from build123d import *

# Parameters (mm, degrees)
BOSS_EXTRUDE1_DEPTH = 5
SKETCH2_W           = 55
SKETCH2_H           = 50
CUT_EXTRUDE1_DEPTH  = 273.349040755
CUT_EXTRUDE2_DEPTH  = 273.349040755
SKETCH4_W           = 30
SKETCH4_H           = 1
CUT_EXTRUDE3_DEPTH  = 273.349040755
CUT_EXTRUDE4_DEPTH  = 273.349040755
CUT_EXTRUDE5_DEPTH  = 273.349040755
CUT_EXTRUDE6_DEPTH  = 273.349040755


with BuildPart() as part:
    # Sketch1 → Boss-Extrude1 (new body)
    with BuildSketch(Plane(origin=(0, 0, 0), x_dir=(1, 0, 0), z_dir=(0, 1, 0))):
        Polygon((0, 0), (0, -43), (30, -43), (30, -48), (0, -48), (0, -73), (90, -73), (90, 257), (-55, 257), (-55, 5), (0, 5), (30, 5), (30, 0), align=None)
    extrude(amount=BOSS_EXTRUDE1_DEPTH)

    # Sketch2 → Cut-Extrude1 (cut, through all)
    with BuildSketch(Plane(origin=(0, 5, 0), x_dir=(1, 0, 0), z_dir=(0, 1, 0))):
        with Locations((-27.5, 232)):
            Rectangle(SKETCH2_W, SKETCH2_H)
    extrude(amount=-CUT_EXTRUDE1_DEPTH, mode=Mode.SUBTRACT)

    # Sketch3 → Cut-Extrude2 (cut, through all)
    with BuildSketch(Plane(origin=(0, 5, 0), x_dir=(1, 0, 0), z_dir=(0, 1, 0))):
        with BuildLine():
            Line((66, 237), (66, 157))
            ThreePointArc((66, 157), (64, 155), (62, 157))
            Line((62, 157), (62, 237))
            ThreePointArc((62, 237), (64, 239), (66, 237))
        make_face()
        with BuildLine():
            Line((66, 127), (66, 47))
            ThreePointArc((66, 47), (64, 45), (62, 47))
            Line((62, 47), (62, 127))
            ThreePointArc((62, 127), (64, 129), (66, 127))
        make_face()
        with BuildLine():
            Line((66, 17), (66, -63))
            ThreePointArc((66, -63), (64, -65), (62, -63))
            Line((62, -63), (62, 17))
            ThreePointArc((62, 17), (64, 19), (66, 17))
        make_face()
        with BuildLine():
            Line((8, 237), (8, 157))
            ThreePointArc((8, 157), (10, 155), (12, 157))
            Line((12, 157), (12, 237))
            ThreePointArc((12, 237), (10, 239), (8, 237))
        make_face()
        with BuildLine():
            Line((8, 127), (8, 47))
            ThreePointArc((8, 47), (10, 45), (12, 47))
            Line((12, 47), (12, 127))
            ThreePointArc((12, 127), (10, 129), (8, 127))
        make_face()
    extrude(amount=-CUT_EXTRUDE2_DEPTH, mode=Mode.SUBTRACT)

    # Sketch4 → Cut-Extrude3 (cut, through all)
    with BuildSketch(Plane(origin=(0, 5, 0), x_dir=(1, 0, 0), z_dir=(0, 1, 0))):
        with Locations((15, -0.5)):
            Rectangle(SKETCH4_W, SKETCH4_H)
        with Locations((15, -42.5)):
            Rectangle(SKETCH4_W, SKETCH4_H)
    extrude(amount=-CUT_EXTRUDE3_DEPTH, mode=Mode.SUBTRACT)

    # Sketch5 → Cut-Extrude4 (cut, through all)
    with BuildSketch(Plane(origin=(0, 5, 0), x_dir=(1, 0, 0), z_dir=(0, 1, 0))):
        with BuildLine():
            Line((6, -19.5), (46, -19.5))
            ThreePointArc((46, -19.5), (48, -21.5), (46, -23.5))
            Line((46, -23.5), (6, -23.5))
            ThreePointArc((6, -23.5), (4, -21.5), (6, -19.5))
        make_face()
        with BuildLine():
            Line((6, -3.5), (46, -3.5))
            ThreePointArc((46, -3.5), (48, -5.5), (46, -7.5))
            Line((46, -7.5), (6, -7.5))
            ThreePointArc((6, -7.5), (4, -5.5), (6, -3.5))
        make_face()
        with BuildLine():
            Line((6, -35.5), (46, -35.5))
            ThreePointArc((46, -35.5), (48, -37.5), (46, -39.5))
            Line((46, -39.5), (6, -39.5))
            ThreePointArc((6, -39.5), (4, -37.5), (6, -35.5))
        make_face()
    extrude(amount=-CUT_EXTRUDE4_DEPTH, mode=Mode.SUBTRACT)

    # Sketch6 → Cut-Extrude5 (cut, through all)
    with BuildSketch(Plane(origin=(0, 5, 0), x_dir=(1, 0, 0), z_dir=(0, 1, 0))):
        with BuildLine():
            Line((-43, 197), (-43, 157))
            ThreePointArc((-43, 157), (-45, 155), (-47, 157))
            Line((-47, 157), (-47, 197))
            ThreePointArc((-47, 197), (-45, 199), (-43, 197))
        make_face()
        with BuildLine():
            Line((-33, 197), (-33, 157))
            ThreePointArc((-33, 157), (-35, 155), (-37, 157))
            Line((-37, 157), (-37, 197))
            ThreePointArc((-37, 197), (-35, 199), (-33, 197))
        make_face()
        with BuildLine():
            Line((-23, 197), (-23, 157))
            ThreePointArc((-23, 157), (-25, 155), (-27, 157))
            Line((-27, 157), (-27, 197))
            ThreePointArc((-27, 197), (-25, 199), (-23, 197))
        make_face()
        with BuildLine():
            Line((-13, 197), (-13, 157))
            ThreePointArc((-13, 157), (-15, 155), (-17, 157))
            Line((-17, 157), (-17, 197))
            ThreePointArc((-17, 197), (-15, 199), (-13, 197))
        make_face()
        with BuildLine():
            Line((-3, 197), (-3, 157))
            ThreePointArc((-3, 157), (-5, 155), (-7, 157))
            Line((-7, 157), (-7, 197))
            ThreePointArc((-7, 197), (-5, 199), (-3, 197))
        make_face()
        with BuildLine():
            Line((-43, 15), (-43, 55))
            ThreePointArc((-43, 55), (-45, 57), (-47, 55))
            Line((-47, 55), (-47, 15))
            ThreePointArc((-47, 15), (-45, 13), (-43, 15))
        make_face()
        with BuildLine():
            Line((-33, 15), (-33, 55))
            ThreePointArc((-33, 55), (-35, 57), (-37, 55))
            Line((-37, 55), (-37, 15))
            ThreePointArc((-37, 15), (-35, 13), (-33, 15))
        make_face()
        with BuildLine():
            Line((-23, 15), (-23, 55))
            ThreePointArc((-23, 55), (-25, 57), (-27, 55))
            Line((-27, 55), (-27, 15))
            ThreePointArc((-27, 15), (-25, 13), (-23, 15))
        make_face()
        with BuildLine():
            Line((-13, 15), (-13, 55))
            ThreePointArc((-13, 55), (-15, 57), (-17, 55))
            Line((-17, 55), (-17, 15))
            ThreePointArc((-17, 15), (-15, 13), (-13, 15))
        make_face()
        with BuildLine():
            Line((-3, 15), (-3, 55))
            ThreePointArc((-3, 55), (-5, 57), (-7, 55))
            Line((-7, 55), (-7, 15))
            ThreePointArc((-7, 15), (-5, 13), (-3, 15))
        make_face()
    extrude(amount=-CUT_EXTRUDE5_DEPTH, mode=Mode.SUBTRACT)

    # Sketch7 → Cut-Extrude6 (cut, through all)
    with BuildSketch(Plane(origin=(0, 5, 0), x_dir=(1, 0, 0), z_dir=(0, 1, 0))):
        with BuildLine():
            Line((-44.604932944, 139), (-5, 139))
            ThreePointArc((-5, 139), (-3, 137), (-5, 135))
            Line((-5, 135), (-44.604932944, 135))
            ThreePointArc((-44.604932944, 135), (-46.604932944, 137), (-44.604932944, 139))
        make_face()
        with BuildLine():
            Line((-44.604932944, 119), (-5, 119))
            ThreePointArc((-5, 119), (-3, 117), (-5, 115))
            Line((-5, 115), (-44.604932944, 115))
            ThreePointArc((-44.604932944, 115), (-46.604932944, 117), (-44.604932944, 119))
        make_face()
        with BuildLine():
            Line((-44.604932944, 99), (-5, 99))
            ThreePointArc((-5, 99), (-3, 97), (-5, 95))
            Line((-5, 95), (-44.604932944, 95))
            ThreePointArc((-44.604932944, 95), (-46.604932944, 97), (-44.604932944, 99))
        make_face()
        with BuildLine():
            Line((-44.604932944, 79), (-5, 79))
            ThreePointArc((-5, 79), (-3, 77), (-5, 75))
            Line((-5, 75), (-44.604932944, 75))
            ThreePointArc((-44.604932944, 75), (-46.604932944, 77), (-44.604932944, 79))
        make_face()
    extrude(amount=-CUT_EXTRUDE6_DEPTH, mode=Mode.SUBTRACT)


solid = part.part
Build history of the part. All positions in model axes, mm. Round coordinates to 2 decimals unless told otherwise and drop trailing zeros. Loops run counter-clockwise (first coordinate to the right, second up) from the corner with the lowest first, then second, coordinate; pieces in that order, holes last. Notation, with made-up numbers: (30.25, 12.25) -> (70.25, 12.25) arc R8 ccw to (70.25, 24.25) -> close; hole circle Ø4 at (69.25, 35.5). An arc over 180 degrees is marked (long way). Use CSV: the item, a comma, the result in double quotes. Start each with the question number.
Q1. Saw through at C-C on z = -219. Give the cut face in (x, y), and give its area (3 significant figures).
Q2. Drill centre lines: L1, parallel to Z at x = -40.5, y = 4.65; L2, parallel to X at y = 1.45, z = -202; L3, parallel to X at y = 0.7, z = 5.5. Where is each one in solid material? Low to high.
Q3. Saw through at A-A on z = 15. Give the cut face in (x, y), and give its area (3 significant figures).
Q4. Saw through at D-D on y = 1.35. Count the separate pieces of the cut face and the enclosed holes in it, and give its area (3 significant figures).
Q5. Flat gauge pins, fed straight in: pin 1 Ø1 at (x, z) = (38.5, -78) entering from -Y; pin 2 Ø2.5 at (y, z) = (3, 30.5) entering from -X; pin 3 Ø1 at (x, y) = (-35.5, 1) entering from +Z; pin 4 Ø2.5 at (x, y) = (-33, 2) entering from -Z. Where does each tip first touch, or does it go through?
Q6. Saw through at B-B on x = 26.5. Give the cut face in (y, z), and give its area (3 significant figures).
Solutions:
1,outline,"(0, 0) -> (8, 0) -> (8, 5) -> (0, 5) -> close; (12, 0) -> (62, 0) -> (62, 5) -> (12, 5) -> close; (66, 0) -> (90, 0) -> (90, 5) -> (66, 5) -> close"
1,area,"410 mm^2"
2,L1,"z = -207 to -139, -135 to -119, -115 to -99, -95 to -79, -75 to -5"
2,L2,"x = -55 to 8, 12 to 62, 66 to 90"
2,L3,"x = 0 to 4, 48 to 62, 66 to 90"
3,outline,"(0, 0) -> (62, 0) -> (62, 5) -> (0, 5) -> close; (66, 0) -> (90, 0) -> (90, 5) -> (66, 5) -> close"
3,area,"430 mm^2"
4,separate pieces,"1"
4,enclosed holes,"22"
4,area,"35,900 mm^2"
5,pin 1,"stops at y = 0"
5,pin 2,"stops at x = 0"
5,pin 3,"stops at z = -5"
5,pin 4,"stops at z = -207"
6,outline,"(0, -257) -> (5, -257) -> (5, -5) -> (0, -5) -> close; (0, 1) -> (5, 1) -> (5, 3.5) -> (0, 3.5) -> close; (0, 7.5) -> (5, 7.5) -> (5, 19.5) -> (0, 19.5) -> close; (0, 23.5) -> (5, 23.5) -> (5, 35.5) -> (0, 35.5) -> close; (0, 39.5) -> (5, 39.5) -> (5, 42) -> (0, 42) -> close; (0, 48) -> (5, 48) -> (5, 73) -> (0, 73) -> close"
6,area,"1,530 mm^2"
